```python
from build123d import *

# Parameters (mm, degrees)
SKETCH1_W           = 139
SKETCH1_H           = 52
SKETCH1_R           = 3.1
SKETCH1_R_2         = 1.6
SKETCH1_R_3         = 3.75
SKETCH1_W_2         = 3.2
SKETCH1_H_2         = 1.9
SKETCH1_W_3         = 2.7
SKETCH1_H_3         = 1.2
BOSS_EXTRUDE1_DEPTH = 3


with BuildPart() as part:
    # Sketch1 → Boss-Extrude1 (new body)
    with BuildSketch(Plane.XY):
        with Locations((69.5, 26)):
            Rectangle(SKETCH1_W, SKETCH1_H)
        with Locations((24.5, 39)):
            Circle(SKETCH1_R, mode=Mode.SUBTRACT)
        with Locations((4, 38)):
            Circle(SKETCH1_R_2, mode=Mode.SUBTRACT)
        with Locations((135, 38)):
            Circle(SKETCH1_R_2, mode=Mode.SUBTRACT)
        with Locations((135, 16)):
            Circle(SKETCH1_R_2, mode=Mode.SUBTRACT)
        with Locations((4, 16)):
            Circle(SKETCH1_R_2, mode=Mode.SUBTRACT)
        with Locations((14.309088021, 21.5)):
            Circle(SKETCH1_R_2, mode=Mode.SUBTRACT)
        with Locations((124, 21.5)):
            Circle(SKETCH1_R_2, mode=Mode.SUBTRACT)
        with Locations((42.5, 39)):
            Circle(SKETCH1_R, mode=Mode.SUBTRACT)
        with Locations((60.5, 39)):
            Circle(SKETCH1_R, mode=Mode.SUBTRACT)
        with Locations((78.5, 39)):
            Circle(SKETCH1_R, mode=Mode.SUBTRACT)
        with Locations((96.5, 39)):
            Circle(SKETCH1_R, mode=Mode.SUBTRACT)
        with Locations((114.5, 39)):
            Circle(SKETCH1_R, mode=Mode.SUBTRACT)
        with Locations((31.5, 15)):
            Circle(SKETCH1_R_3, mode=Mode.SUBTRACT)
        with Locations((31.5, 7.3)):
            Rectangle(SKETCH1_W_2, SKETCH1_H_2, mode=Mode.SUBTRACT)
        with Locations((24.5, 33)):
            Rectangle(SKETCH1_W_3, SKETCH1_H_3, mode=Mode.SUBTRACT)
        with Locations((42.5, 33)):
            Rectangle(SKETCH1_W_3, SKETCH1_H_3, mode=Mode.SUBTRACT)
        with Locations((60.5, 33)):
            Rectangle(SKETCH1_W_3, SKETCH1_H_3, mode=Mode.SUBTRACT)
        with Locations((78.5, 33)):
            Rectangle(SKETCH1_W_3, SKETCH1_H_3, mode=Mode.SUBTRACT)
        with Locations((96.5, 33)):
            Rectangle(SKETCH1_W_3, SKETCH1_H_3, mode=Mode.SUBTRACT)
        with Locations((114.5, 33)):
            Rectangle(SKETCH1_W_3, SKETCH1_H_3, mode=Mode.SUBTRACT)
        with BuildLine():
            Line((67.436628972, 12.05), (71.563371028, 12.05))
            ThreePointArc((71.563371028, 12.05), (73.1, 15), (71.563371028, 17.95))
            Line((71.563371028, 17.95), (67.436628972, 17.95))
            ThreePointArc((67.436628972, 17.95), (65.9, 15), (67.436628972, 12.05))
        make_face(mode=Mode.SUBTRACT)
    extrude(amount=BOSS_EXTRUDE1_DEPTH)


solid = part.part
```
For this review, take the finished solid that the model builds, in its own axes (mm). A direction names the side the tool comes from. Coordinates: 2 decimals unless noted, no trailing zeros. Loops run counter-clockwise (first coordinate to the right, second up) from the corner with the lowest first, then second, coordinate; pieces in that order, holes last. Notation, with made-up numbers: (10.25, -2.75) -> (23.25, -2.75) arc R23 ccw to (23.25, 29.25) -> close; hole circle Ø10 at (21, 36.5). An arc over 180 degrees is marked (long way). Return JSON: item names as keys, results as strings. Group by question number.
(1) For pin 1 Ø1.9 at (x, y) = (135, 16) entering from +Z, flat-tipped, find the tip position at first contact; note if it passes through.
(2) Consider section A-A, the plane x = 4. Give the boundary of the cut face in (y, z).
(3) Mouldability with a two-part tool opening along Y and no side actions: class faces 3 (the flat face through (69, 26, 0)), 4 (the cylindrical face through (136.48, 37.39, 1.48)), 5 (the flat face through (24, 32.4, 1)) as pulls with the +Y half, pulls with the -Y half, needs draft (parallel to the pull), parting line crosses it, or undercut.
(4) To check wall thickness, follow L1, parallel to Y at x = 114.5, z = 0.6; L2, parallel to Y at x = 135, z = 1.55; L3, parallel to X at y = 17, z = 0.15. State the ranges of each line that lie inside material, in increasing order.
(5) Consider section C-C, the plane x = 124. Give the boundary of the cut face in (y, z).
(6) Consider section D-D, the plane z = 1.55. Count the separate pieces of the cut face and the enclosed holes in it, plus the area to 3 significant figures.
(7) Consider section B-B, the plane y = 21.5. Give the boundary of the cut face in (x, z), plus the area to 3 significant figures.
(8) Tool access review of faces 1 (the flat face through (69, 26, 3)), 2 (the flat face through (70, 17.95, 1)): name each direction out of +Z, -Z, +X, -X, +Y, -Y from which nothing blocks a thin tool from reaching the whole face with its end or side.
Results below:
{
 "1": {"pin 1": "passes through"},
 "2": {"outline": "(0, 0) -> (14.4, 0) -> (14.4, 3) -> (0, 3) -> close; (17.6, 0) -> (36.4, 0) -> (36.4, 3) -> (17.6, 3) -> close; (39.6, 0) -> (52, 0) -> (52, 3) -> (39.6, 3) -> close"},
 "3": {"face 3": "needs draft", "face 4": "undercut", "face 5": "undercut"},
 "4": {"L1": "y = 0 to 32.4, 33.6 to 35.9, 42.1 to 52", "L2": "y = 0 to 14.4, 17.6 to 36.4, 39.6 to 52", "L3": "x = 0 to 2.75, 5.25 to 28.33, 34.67 to 66.51, 72.49 to 133.75, 136.25 to 139"},
 "5": {"outline": "(0, 0) -> (19.9, 0) -> (19.9, 3) -> (0, 3) -> close; (23.1, 0) -> (52, 0) -> (52, 3) -> (23.1, 3) -> close"},
 "6": {"separate pieces": "1", "enclosed holes": "21", "area": "6,890 mm2"},
 "7": {"outline": "(0, 0) -> (12.71, 0) -> (12.71, 3) -> (0, 3) -> close; (15.91, 0) -> (122.4, 0) -> (122.4, 3) -> (15.91, 3) -> close; (125.6, 0) -> (139, 0) -> (139, 3) -> (125.6, 3) -> close", "area": "398 mm2"},
 "8": {"face 1": "+Z, +X, -X, +Y, -Y", "face 2": "+Z, -Z"}
}
